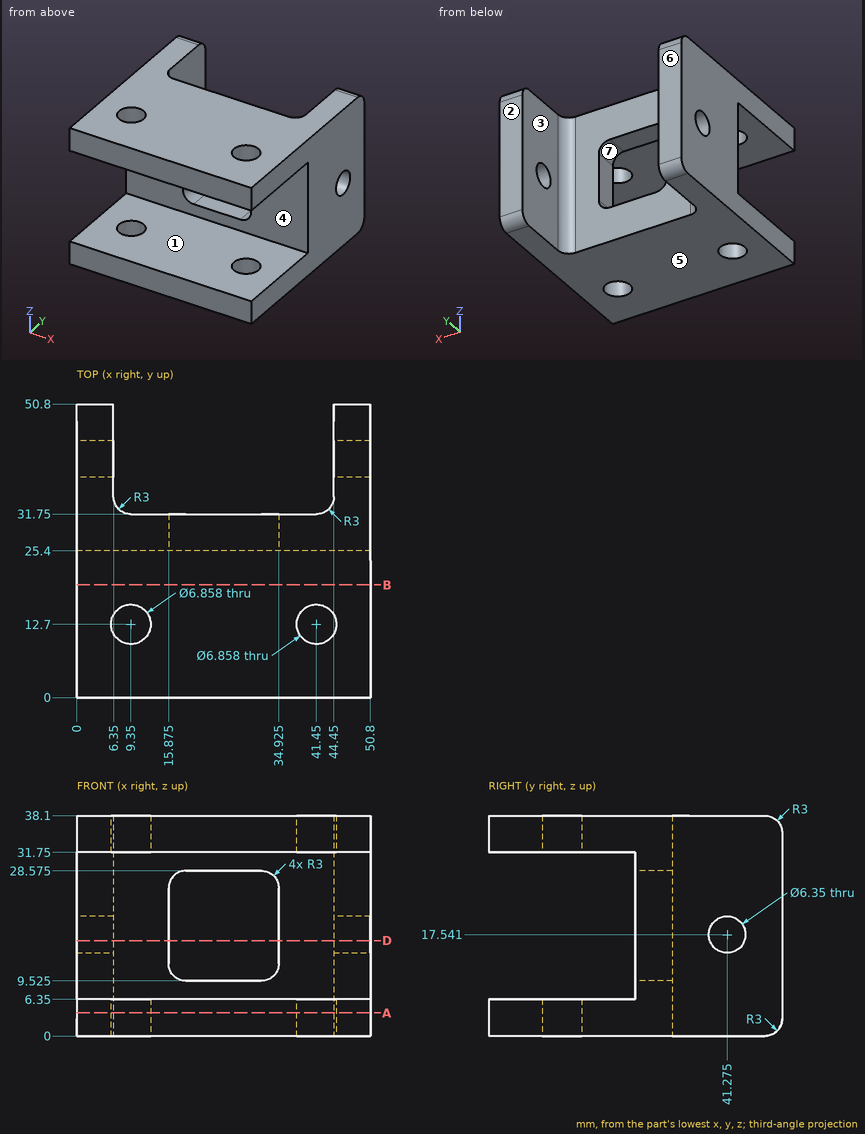
Input: dimensioned drawing with shaded views. Units: mm. Origin: part minimum x, y, z. A direction names the side the tool comes from. Give positions to 0.01 mm unless a question says otherwise; leave off trailing zeros. Loops run counter-clockwise (first coordinate to the right, second up) from the corner with the lowest first, then second, coordinate; pieces in that order, holes last. Notation, with made-up numbers: (87.25, 27.25) -> (143.25, 27.25) arc R24 cw to (143.25, 50.25) -> close; hole circle Ø2 at (62, -16). An arc over 180 degrees is marked (long way). Use a Markdown table: item, result.
Q1. Section query B-B, the plane y = 19.5. Return the cut outline in (x, z), plus the area to 3 significant figures.
Entries:
| item | result |
|---|---|
| outline | (0, 0) -> (50.8, 0) -> (50.8, 6.35) -> (0, 6.35) -> close; (0, 31.75) -> (50.8, 31.75) -> (50.8, 38.1) -> (0, 38.1) -> close |
| area | 645 mm² |
Q2. Ray query, probe 1 along Z at (x, y) = (43, 20.5); probe 2 along X at (y, z) = (12, 3); probe 3 along X at (y, z) = (44, 15.5). Return the intervals inside material, ascending. Write a range as from..to.
Entries:
| item | result |
|---|---|
| probe 1 | z = 0..6.35, 31.75..38.1 |
| probe 2 | x = 0..5.99, 12.71..38.09, 44.81..50.8 |
| probe 3 | x = 0..6.35, 44.45..50.8 |
Q3. Section query D-D, the plane z = 16.5. State how many separate pieces and enclosed holes the cut face has, plus the area to 3 significant figures.
Entries:
| item | result |
|---|---|
| separate pieces | 4 |
| enclosed holes | 0 |
| area | 371 mm² |
Q4. Access query for the marked faces 1, 2 and 3. Directions: +Z, -Z, +X, -X, +Y, -Y. A direction counts if a zero-diameter tool reaches every point of the face in a straight line with its end or side. Return the directions, or none.
Entries:
| item | result |
|---|---|
| face 1 | +X, -X, -Y |
| face 2 | +Z, -Z, +X, -X, +Y |
| face 3 | +Z, -Z, +Y |
Q5. Pull-direction query (Z, two-part tool) for the marked faces 4, 5, 6 and 7; classes: pulls with the +Z half, pulls with the -Z half, needs draft (parallel to the pull), parting line crosses it, or undercut.
Entries:
| item | result |
|---|---|
| face 4 | undercut |
| face 5 | pulls with the -Z half |
| face 6 | needs draft |
| face 7 | undercut |
Q6. First-contact query: P1, Ø4, axis at y = 41.28, z = 17.54, coming from the +X side; P2, Ø8, axis at x = 10, z = 12.5, coming from the -Y side. Flat tips, straight axial feed; report the tip coordinate or a pass-through.
Entries:
| item | result |
|---|---|
| P1 | passes through |
| P2 | stops at y = 25.4 |
Q7. Section query A-A, the plane z = 4. Return the cut outline in (x, y), plus the area to 4 significant figures.
Entries:
| item | result |
|---|---|
| outline | (0, 0) -> (50.8, 0) -> (50.8, 50.8) -> (44.45, 50.8) -> (44.45, 34.75) arc R3 cw to (41.45, 31.75) -> (9.35, 31.75) arc R3 cw to (6.35, 34.75) -> (6.35, 50.8) -> (0, 50.8) -> close; hole circle Ø6.86 at (9.35, 12.7); hole circle Ø6.86 at (41.45, 12.7) |
| area | 1,785 mm² |
